```python
from build123d import *

# Parameters (mm, degrees)
SKETCH_W        = 60
SKETCH_H        = 40
PAD_DEPTH       = 10
PAD001_DEPTH    = 20
PAD002_DEPTH    = 9
SKETCH003_R     = 5
POCKET_DEPTH    = 39.001
POCKET001_DEPTH = 40.001
POCKET002_DEPTH = 197.61763
SKETCH006_W     = 30
SKETCH006_H     = 3
POCKET003_DEPTH = 40.001


with BuildPart() as part:
    # Sketch → Pad (new body)
    with BuildSketch(Plane.XY):
        Rectangle(SKETCH_W, SKETCH_H)
    extrude(amount=PAD_DEPTH)

    # Sketch001 → Pad001 (join, symmetric)
    with BuildSketch(Plane.XZ):
        with BuildLine():
            Line((20, 25), (20, 10))
            Line((20, 10), (-20, 10))
            Line((-20, 10), (-20, 25))
            ThreePointArc((20, 25), (0, 45), (-20, 25))
        make_face()
    extrude(amount=PAD001_DEPTH, both=True)

    # Sketch002 → Pad002 (join, symmetric)
    with BuildSketch(Plane.YZ):
        with BuildLine():
            Line((-10, 23), (-10, 50))
            ThreePointArc((10, 50), (0, 60), (-10, 50))
            Line((10, 50), (10, 23))
            Line((10, 23), (-10, 23))
        make_face()
    extrude(amount=PAD002_DEPTH, both=True)

    # Sketch003 (on Face15 of Pad002) → Pocket (cut, through all)
    with BuildSketch(Plane.YZ.offset(9)):
        with Locations((0, 50)):
            Circle(SKETCH003_R)
    extrude(amount=-POCKET_DEPTH, mode=Mode.SUBTRACT)

    # Sketch004 (on Face12 of Pocket) → Pocket001 (cut, through all)
    with BuildSketch(Plane.XZ.offset(20)):
        with BuildLine():
            ThreePointArc((-2, 37.845233), (0, 12), (2, 37.845233))
            Line((2, 70), (2, 37.845233))
            Line((-2, 70), (2, 70))
            Line((-2, 37.845233), (-2, 70))
        make_face()
    extrude(amount=-POCKET001_DEPTH, mode=Mode.SUBTRACT)

    # Sketch005 (on Face7 of Pocket001) → Pocket002 (cut, through all)
    with BuildSketch(Plane.XY.offset(10)):
        with BuildLine():
            ThreePointArc((27, 12), (25, 14), (23, 12))
            Line((23, 12), (23, -12))
            ThreePointArc((23, -12), (25, -14), (27, -12))
            Line((27, 12), (27, -12))
        make_face()
    pocket002 = extrude(amount=-POCKET002_DEPTH, mode=Mode.SUBTRACT)

    # Mirrored: Pocket002 across Sketch005 V_Axis
    add(pocket002.mirror(Plane(origin=(0, 0, 10), x_dir=(0, 0, 1), z_dir=(1, 0, 0))), mode=Mode.SUBTRACT)

    # Sketch006 (on Face8 of Mirrored) → Pocket003 (cut, through all)
    with BuildSketch(Plane.XZ.offset(20)):
        with Locations((0, 1.5)):
            Rectangle(SKETCH006_W, SKETCH006_H)
    extrude(amount=-POCKET003_DEPTH, mode=Mode.SUBTRACT)


solid = part.part
```
CAD build for the part. Positions are in the model's coordinates, mm. A direction names the side the tool comes from. Round coordinates to 2 decimals unless told otherwise and drop trailing zeros. Loops run counter-clockwise (first coordinate to the right, second up) from the corner with the lowest first, then second, coordinate; pieces in that order, holes last. Notation, with made-up numbers: (49.5, -38) - (73.5, -38) arc R12 cw to (73.5, -26) - close; hole circle Ø3 at (66.25, 33.5). An arc over 180 degrees is marked (long way). Return JSON: item names as keys, results as strings. Group by question number.
Q1. Band-saw the part on C-C on z = 13.5. Give the cut face in (x, y).
Q2. Tool access for faces 1 (the face through (25, 14, 5)), 2 (the face through (0, 0, 3)), 3 (the face through (-5, 10, 47)), 4 (the face through (6, -10, 47)), 5 (the face through (9, 0.1, 55.4)): list every direction of +Z, -Z, +X, -X, +Y, -Y with a clear straight run to the whole face (end or side of a thin tool).
Q3. Two-plate mould, pull along Y, no slides. Class faces 6 (the face through (6, -20, 12)), 7 (the face through (27, 0, 5)), 8 (the face through (-2, 0, 44)): +Y half, -Y half, draft (parallel to the pull), parting line (faces both ways), or undercut.
Q4. Flat gauge pins, fed straight in: pin 1 Ø11 at (y, z) = (-5.5, 49.5) entering from +X; pin 2 Ø13.5 at (y, z) = (3, 54) entering from -X; pin 3 Ø2 at (x, z) = (6.5, 48) entering from -Y. Where does each tip first touch, or does it go through?
Q5. Band-saw the part on A-A on y = 8. Give the cut face in (x, z), plus the area to 3 significant figures.
Q6. Drill centre lines: line 1 along X through (y, z) = (3, 7); line 2 along X through (y, z) = (17.5, 24.5); line 3 along Z through (x, y) = (-5.5, 0). Where is each one in solid material? Low to high. Write a range as [from, to].
Q7. Band-saw the part on B-B on x = -25. Give the cut face in (y, z), plus the area to 3 significant figures.
Q8. Band-saw the part on D-D on y = 15. Give the cut face in (x, z).
Solutions:
{
 "1": {"outline": "(-20, -20) - (-6.06, -20) - (-6.06, 20) - (-20, 20) - close; (6.06, -20) - (20, -20) - (20, 20) - (6.06, 20) - close"},
 "2": {"face 1": "+Z, -Z", "face 2": "-Z, +Y, -Y", "face 3": "+Z, -X, +Y", "face 4": "+Z, +X, -Y", "face 5": "+Z, +X, +Y, -Y"},
 "3": {"face 6": "-Y half", "face 7": "undercut", "face 8": "draft"},
 "4": {"pin 1": "stops at x = 9", "pin 2": "stops at x = -9", "pin 3": "stops at y = -10"},
 "5": {"outline": "(-30, 0) - (-27, 0) - (-27, 10) - (-30, 10) - close; (-23, 0) - (-15, 0) - (-15, 3) - (15, 3) - (15, 0) - (23, 0) - (23, 10) - (20, 10) - (20, 25) arc R20 ccw to (9, 42.86) - (9, 56) - (2, 56) - (2, 37.85) arc R13 cw (long way) to (-2, 37.85) - (-2, 56) - (-9, 56) - (-9, 42.86) arc R20 ccw to (-20, 25) - (-20, 10) - (-23, 10) - close; (27, 0) - (30, 0) - (30, 10) - (27, 10) - close", "area": "1,270 mm^2"},
 "6": {"line 1": "x = [-30, -27], [-23, 23], [27, 30]", "line 2": "x = [-20, -12.99], [12.99, 20]", "line 3": "z = [3, 13.22], [36.78, 45], [55, 60]"},
 "7": {"outline": "(-20, 0) - (-14, 0) - (-14, 10) - (-20, 10) - close; (14, 0) - (20, 0) - (20, 10) - (14, 10) - close", "area": "120 mm^2"},
 "8": {"outline": "(-30, 0) - (-15, 0) - (-15, 3) - (15, 3) - (15, 0) - (30, 0) - (30, 10) - (20, 10) - (20, 25) arc R20 ccw to (2, 44.9) - (2, 37.85) arc R13 cw (long way) to (-2, 37.85) - (-2, 44.9) arc R20 ccw to (-20, 25) - (-20, 10) - (-30, 10) - close"}
}
